Autodesk Fusion 360 part; units mm, degrees
sketch "Sketch1" plane through (0, 0, 0) normal (0, 0, 1) x (1, 0, 0)
  line L0 (3.309, 32.844) -> (14.9188, 32.844)
  line L1 (26.2752, -6.3858) -> (26.2752, -22.9908)
  arc A0 (16.422, -22.9908) -> (26.2752, -22.9908) centre (21.3486, -22.9908) ccw
  line L2 (16.422, -22.9908) -> (16.422, -11.4954)
  line L3 (5.3015, -11.7323) -> (18.4305, -27.6914)
  arc A1 (15.6271, -36.4434) -> (18.4305, -27.6914) centre (14.2091, -31.1642) ccw
  line L4 (15.6271, -36.4434) -> (-3.6897, -17.1266)
  line L5 (-6.5756, -10.1593) -> (-6.5756, 1.4585)
  line L6 (-3.2683, 9.443) -> (-3.7397, 8.9716)
  line L7 (0.1079, 18.3592) -> (0.0246, 29.5352)
  line L8 (18.2032, 29.5596) -> (18.2032, 15.961)
  line L9 (19.5902, 10.0856) -> (24.8883, -0.5105)
  arc A2 (-3.2683, 9.443) -> (-6.5756, 1.4585) centre (4.7161, 1.4585) ccw
  line L10 (9.8532, -4.9266) -> (7.8379, -4.9266)
  line L11 (4.5535, -8.211) -> (4.5535, -9.6457)
  arc A3 (7.8379, -4.9266) -> (4.5535, -8.211) centre (7.8379, -8.211) ccw
  arc A4 (4.5535, -9.6457) -> (5.3015, -11.7323) centre (7.8379, -9.6457) ccw
  arc A5 (16.422, -11.4954) -> (9.8532, -4.9266) centre (9.8532, -11.4954) ccw
  arc A6 (-6.5756, -10.1593) -> (-3.6897, -17.1266) centre (3.2776, -10.1593) ccw
  arc A7 (26.2752, -6.3858) -> (24.8883, -0.5105) centre (13.1376, -6.3858) ccw
  arc A8 (18.2032, 15.961) -> (19.5902, 10.0856) centre (31.3409, 15.961) ccw
  arc A9 (-3.7397, 8.9716) -> (0.1079, 18.3592) centre (-13.0294, 18.2613) ccw
  arc A10 (3.309, 32.844) -> (0.0246, 29.5352) centre (3.309, 29.5596) ccw
  arc A11 (18.2032, 29.5596) -> (14.9188, 32.844) centre (14.9188, 29.5596) ccw
  arc A12 (-1.147, 7.3217) -> (-3.5756, 1.4585) centre (4.7161, 1.4585) ccw
  line L12 (-3.5756, -10.1593) -> (-3.5756, 1.4585)
  arc A13 (-3.5756, -10.1593) -> (-1.5683, -15.0053) centre (3.2776, -10.1593) ccw
  line L13 (16.1333, -32.7069) -> (-1.5683, -15.0053)
  arc A14 (16.1333, -32.7069) -> (16.1137, -29.5973) centre (14.2091, -31.1642) ccw
  line L14 (2.9847, -13.6383) -> (16.1137, -29.5973)
  arc A15 (1.5535, -9.6457) -> (2.9847, -13.6383) centre (7.8379, -9.6457) ccw
  line L15 (1.5535, -8.211) -> (1.5535, -9.6457)
  arc A16 (7.8379, -1.9266) -> (1.5535, -8.211) centre (7.8379, -8.211) ccw
  line L16 (9.8532, -1.9266) -> (7.8379, -1.9266)
  arc A17 (19.422, -11.4954) -> (9.8532, -1.9266) centre (9.8532, -11.4954) ccw
  line L17 (19.422, -22.9908) -> (19.422, -11.4954)
  arc A18 (19.422, -22.9908) -> (23.2752, -22.9908) centre (21.3486, -22.9908) ccw
  line L18 (23.2752, -6.3858) -> (23.2752, -22.9908)
  arc A19 (23.2752, -6.3858) -> (22.205, -1.8521) centre (13.1376, -6.3858) ccw
  line L19 (16.9069, 8.744) -> (22.205, -1.8521)
  arc A20 (15.2032, 15.961) -> (16.9069, 8.744) centre (31.3409, 15.961) ccw
  line L20 (15.2032, 29.5596) -> (15.2032, 15.961)
  arc A21 (15.2032, 29.5596) -> (14.9188, 29.844) centre (14.9188, 29.5596) ccw
  line L21 (3.309, 29.844) -> (14.9188, 29.844)
  arc A22 (3.309, 29.844) -> (3.0246, 29.5575) centre (3.309, 29.5596) ccw
  line L22 (3.1078, 18.3815) -> (3.0246, 29.5575)
  arc A23 (-0.8215, 7.7071) -> (3.1078, 18.3815) centre (-13.0294, 18.2613) ccw
  arc A24 (-1.147, 7.3217) -> (-0.8215, 7.7071) centre (-3.2683, 9.443) ccw
  dimension "d13" = 3
extrude "Extrude1" add sketch "Sketch1" along normal blind 15
sketch "Sketch2" plane through (0, 0, 0) normal (0, 1, 0) x (1, 0, 0)
Model file for the job. Use its own axes, mm. A direction names the side the tool comes from. Give positions to 0.01 mm unless a question says otherwise; leave off trailing zeros. Write each loop counter-clockwise with the first axis right and the second up, starting at its lowest first coordinate (ties: lowest second). Pieces come first, ordered by that corner, then holes. Notation, with made-up numbers: (74.5, 20.25) - (126.5, 20.25) arc R14 ccw to (126.5, 42.25) - close; hole circle Ø4 at (-40, 32). An arc over 180 degrees is marked (long way). Answer as CSV lines item,"result".
1. Pin check, flat tips, straight feed: pin 1 (2 mm diameter, centred on x = 13.5, z = 7, fed in from -Y); pin 2 (5 mm diameter, centred on y = 15.5, z = 9, fed in from -X); pin 3 (9 mm diameter, centred on y = -19, z = 9.5, fed in from -X). Stop position of each tip, or through.
Responses:
pin 1,"stops at y = -35.32"
pin 2,"stops at x = -0.99"
pin 3,"stops at x = -5.57"
2. Two-plate mould, pull along X, no slides. Class faces 1 (the face through (1.554, -9, 7)), 2 (the face through (17.216, 31.907, 7.395)), 3 (the face through (-5.805, -13.98, 7.395)): +X half, -X half, draft (parallel to the pull), parting line (faces both ways), or undercut.
Responses:
face 1,"undercut"
face 2,"+X half"
face 3,"-X half"
3. Band-saw the part on B-B (y = -26.5). Write the cut outline in (x, z), and give its area (3 significant figures).
Responses:
outline,"(5.68, 0) - (9.93, 0) - (9.93, 15) - (5.68, 15) - close; (13.57, 0) - (17.45, 0) - (17.45, 15) - (13.57, 15) - close; (17.89, 0) - (24.81, 0) - (24.81, 15) - (17.89, 15) - close"
area,"226 mm2"
4. Drill centre lines: L1, parallel to X at y = -23.5, z = 2.5; L2, parallel to Y at x = 10.5, z = 10.75; L3, parallel to Y at x = 14.5, z = 2.25. Where is each one in solid material? Low to high. Write a range as [from, to].
Responses:
L1,"x = [2.68, 6.93], [11.1, 14.98], [16.45, 19.49], [23.21, 26.25]"
L2,"y = [-31.32, -27.07], [-22.77, -18.05], [-4.96, -1.95], [29.84, 32.84]"
L3,"y = [-35.32, -31.07], [-27.64, -22.91], [-6.85, -3.13], [29.84, 32.84]"
5. Band-saw the part on C-C (y = -3.5). Write the cut outline in (x, z), and give its area (3 significant figures).
Responses:
outline,"(-6.58, 0) - (-3.58, 0) - (-3.58, 15) - (-6.58, 15) - close; (3.68, 0) - (15.11, 0) - (15.11, 15) - (3.68, 15) - close; (22.86, 0) - (25.95, 0) - (25.95, 15) - (22.86, 15) - close"
area,"263 mm2"
6. Band-saw the part on A-A (x = 13.5). Write the cut outline in (y, z).
Responses:
outline,"(-34.32, 0) - (-30.07, 0) - (-30.07, 15) - (-34.32, 15) - close; (-26.42, 0) - (-21.7, 0) - (-21.7, 15) - (-26.42, 15) - close; (-6.03, 0) - (-2.65, 0) - (-2.65, 15) - (-6.03, 15) - close; (29.84, 0) - (32.84, 0) - (32.84, 15) - (29.84, 15) - close"
7. 3-axis set-ups, long thin cutter, end or side, ignore diameter. For faces 4 (the face through (18.565, 12.901, 7.395)), 5 (the face through (23.275, -15, 7)): which of +Z, -Z, +X, -X, +Y, -Y reach the whole face in a straight line?
Responses:
face 4,"+Z, -Z, +X, +Y"
face 5,"+Z, -Z"
